Work out the finished part from the listing and answer in its coordinate system (mm). Face numbers are marked on the shaded views. Round coordinates to 2 decimals unless told otherwise and drop trailing zeros. Order: outer loops, then holes, each group sorted by start corner. A loop starts at its lowest first (then second) coordinate and runs counter-clockwise, first axis right, second up. Notation, with made-up numbers: (32.5, 43) -> (90.5, 43) arc R22 cw to (90.5, 65) -> close; hole circle Ø6 at (-17.5, -0.75). An arc over 180 degrees is marked (long way). Use a Markdown table: item, result. Add a question column.
Item 1: A cutting plane is placed at A-A, the plane y = 5. Determine the outline of the cut face in (x, z).
Item 2: For a pull along Z with two mould halves and no side action, classify the marked faces 1 and 2 as +Z half, -Z half, draft (parallel to the pull), parting line (faces both ways), or undercut.
Item 3: Find the intervals of material crossed by L1, parallel to Z at x = 18, y = 5; L2, parallel to Z at x = 4, y = 5; L3, parallel to Y at x = 34.5, z = 26, in increasing order. Write a range as [from, to].
Item 4: A cutting plane is placed at D-D, the plane x = 11. Determine the outline of the cut face in (y, z).
Item 5: Flat-ended cylindrical pins translate along their axes: P1, Ø1.5, axis at x = 51.5, y = 2.5, coming from the -Z side; P2, Ø2, axis at y = 4, z = 55.5, coming from the +X side. Find the tip coordinate at first contact, or state that the pin passes through.
Item 6: A cutting plane is placed at B-B, the plane x = 61. Determine the outline of the cut face in (y, z), plus the area to 3 significant figures.
Item 7: A cutting plane is placed at C-C, the plane z = 49.5. Determine the outline of the cut face in (x, y), plus the area to 3 significant figures.
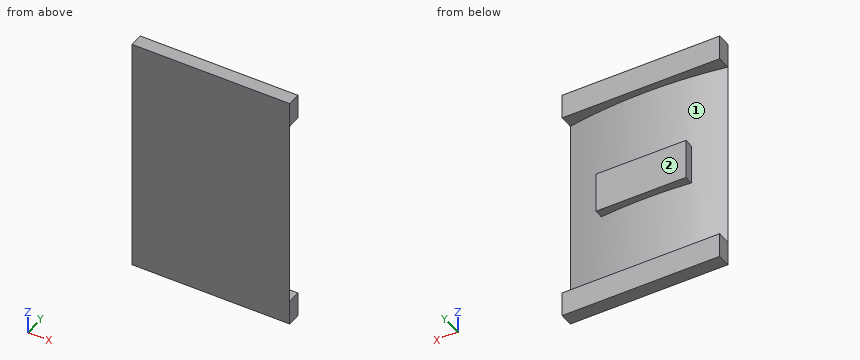
from build123d import *

# Parameters (mm, degrees)
F1_DEPTH = 107
F2_W     = 70
F2_H     = 11
F2_W_2   = 40
F2_H_2   = 18
F3_DEPTH = 6


with BuildPart() as f1:
    # F0 (on Top) → F1 (new body)
    with BuildSketch(Plane.XY):
        with BuildLine():
            Line((0, 0), (70, 0))
            ThreePointArc((70, 0), (35, 3), (0, 0))
        make_face()
    extrude(amount=F1_DEPTH)

    # F2 (on face) → F3 (join)
    with BuildSketch(Plane.XZ):
        with Locations((35, 101.5)):
            Rectangle(F2_W, F2_H)
        with Locations((35, 53.5)):
            Rectangle(F2_W_2, F2_H_2)
        with Locations((35, 5.5)):
            Rectangle(F2_W, F2_H)
    extrude(amount=-F3_DEPTH)


solid = f1.part
Reported:
| question | item | result |
|---|---|---|
| 1 | outline | (0, 0) -> (70, 0) -> (70, 11) -> (0, 11) -> close; (0, 96) -> (70, 96) -> (70, 107) -> (0, 107) -> close; (15, 44.5) -> (55, 44.5) -> (55, 62.5) -> (15, 62.5) -> close |
| 2 | face 1 | undercut |
| 2 | face 2 | draft |
| 3 | L1 | [0, 11], [44.5, 62.5], [96, 107] |
| 3 | L2 | [0, 11], [96, 107] |
| 3 | L3 | [0, 3] |
| 4 | outline | (0, 0) -> (6, 0) -> (6, 11) -> (1.59, 11) -> (1.59, 96) -> (6, 96) -> (6, 107) -> (0, 107) -> close |
| 5 | P1 | z = 0 |
| 5 | P2 | x = 55 |
| 6 | outline | (0, 0) -> (6, 0) -> (6, 11) -> (1.35, 11) -> (1.35, 96) -> (6, 96) -> (6, 107) -> (0, 107) -> close |
| 6 | area | 247 mm² |
| 7 | outline | (0, 0) -> (70, 0) arc R205.67 ccw to (55, 2.03) -> (55, 6) -> (15, 6) -> (15, 2.03) arc R205.67 ccw to start |
| 7 | area | 273 mm² |
